Here's how the part is built. I have some questions about the finished solid (model axes, mm). A direction names the side the tool comes from. Coordinates: 2 decimals unless noted, no trailing zeros. Loops run counter-clockwise (first coordinate to the right, second up) from the corner with the lowest first, then second, coordinate; pieces in that order, holes last. Notation, with made-up numbers: (32, 13.5) -> (79, 13.5) arc R11 cw to (79, 26.5) -> close; hole circle Ø9 at (-8, 36.25). An arc over 180 degrees is marked (long way). Answer as a JSON object with one key per item and string values. Group by question number.
1) I want a section at B-B (x = -16). Write out the boundary of the cut face in (y, z).
2) I want a section at A-A (z = 8.5). Write out the boundary of the cut face in (x, y), then the cut area to 3 significant figures.
3) Which directions (+Z, -Z, +X, -X, +Y, -Y) give clear straight access to the entire face, cutting with the end or side of a thin tool? Please do faces 1 (the flat face through (51.619, 2, 5)), 2 (the cylindrical face through (44.05, 1.528, 36.896)).
4) I'm going to push a flat-ended pin straight in: pin 1 (1.9 mm diameter, centred on x = -45.37, z = 38.9, fed in from -Y). Where does the tip first touch, or does it pass through?
5) I want a section at C-C (y = 0.7). Write out the boundary of the cut face in (x, z), then the cut area to 3 significant figures.
6) I need wall thicknesses on probe 1 along X at (y, z) = (2.5, 6.5); probe 2 along Z at (x, y) = (-1, 0.2); probe 3 along Z at (x, y) = (42.5, 1.25). Which ranges of each line are inside material? Lowest first, please. Write a range as [from, to].
7) If we mould it in two halves opening along Z, with no side actions, what happens to faces 3 (the cylindrical face through (40.54, 1.53, -34.79)), 4 (the flat face through (-6, 2, -45.601)), 5 (the flat face through (1, 2, 44.239)), 6 (the flat face through (12, 0, 39))? For each: +Z half, -Z half, draft (parallel to the pull), parting line (faces both ways), or undercut.
```python
from build123d import *

# Parameters (mm, degrees)
SKETCH1_R           = 1.549999996
SKETCH1_R_2         = 1.549999999
SKETCH1_R_3         = 1.550000006
SKETCH1_R_4         = 1.55
BOSS_EXTRUDE1_DEPTH = 3.1


with BuildPart() as part:
    # Sketch1 → Boss-Extrude1 (new body)
    with BuildSketch(Plane(origin=(0, 0, 0), x_dir=(1, 0, 0), z_dir=(0, 1, 0))):
        with BuildLine():
            Line((-39.710740333, 45.601389456), (28.739259425, 45.601389477))
            ThreePointArc((28.739259425, 45.601389477), (44.917862489, 38.899992874), (51.619259444, 22.721389957))
            Line((51.619259444, 22.721389957), (51.619259444, -33.910608927))
            ThreePointArc((51.619259444, -33.910608927), (48.176648434, -41.250850634), (40.639804947, -44.238610519))
            Line((40.639804947, -44.238610519), (-39.710740094, -44.238610544))
            ThreePointArc((-39.710740094, -44.238610544), (-47.488914725, -41.01678516), (-50.710740163, -33.23861055))
            Line((-50.710740163, -33.23861055), (-50.710740163, 34.601389583))
            ThreePointArc((-50.710740163, 34.601389583), (-47.488914793, 42.379564056), (-39.710740333, 45.601389456))
        make_face()
        with Locations(Location((-45.367594445, 40.258243716, 0), (0, 0, 90))):
            Circle(SKETCH1_R, mode=Mode.SUBTRACT)
        with Locations(Location((-45.367594389, -38.895464809, 0), (0, 0, 90))):
            Circle(SKETCH1_R_2, mode=Mode.SUBTRACT)
        with Locations(Location((46.094048666, -39.090808696, 0), (0, 0, 90))):
            Circle(SKETCH1_R_3, mode=Mode.SUBTRACT)
        with Locations(Location((42.796542168, 36.778672508, 0), (0, 0, 90))):
            Circle(SKETCH1_R_4, mode=Mode.SUBTRACT)
        with BuildLine():
            Line((-39.710740331, 39.601389456), (28.739259427, 39.601389477))
            ThreePointArc((28.739259427, 39.601389477), (40.675221825, 34.657352163), (45.619259444, 22.721389891))
            Line((45.619259444, 22.721389891), (45.619259444, -33.691417556))
            ThreePointArc((45.619259444, -33.691417556), (44.011448898, -36.930766758), (40.639804981, -38.238610519))
            Line((40.639804981, -38.238610519), (-39.710740095, -38.238610544))
            ThreePointArc((-39.710740095, -38.238610544), (-43.246274043, -36.774144468), (-44.710740163, -33.238610539))
            Line((-44.710740163, -33.238610539), (-44.710740163, 34.601389583))
            ThreePointArc((-44.710740163, 34.601389583), (-43.246274105, 38.136923369), (-39.710740331, 39.601389456))
        make_face(mode=Mode.SUBTRACT)
    extrude(amount=BOSS_EXTRUDE1_DEPTH)


solid = part.part
```
Determined:
{
 "1": {"outline": "(0, -45.6) -> (3.1, -45.6) -> (3.1, -39.6) -> (0, -39.6) -> close; (0, 38.24) -> (3.1, 38.24) -> (3.1, 44.24) -> (0, 44.24) -> close"},
 "2": {"outline": "(-50.71, 0) -> (-44.71, 0) -> (-44.71, 3.1) -> (-50.71, 3.1) -> close; (45.62, 0) -> (51.62, 0) -> (51.62, 3.1) -> (45.62, 3.1) -> close", "area": "37.2 mm^2"},
 "3": {"face 1": "+Z, -Z, +X, +Y, -Y", "face 2": "+Y, -Y"},
 "4": {"pin 1": "through"},
 "5": {"outline": "(-50.71, -34.6) arc R11 ccw to (-39.71, -45.6) -> (28.74, -45.6) arc R22.88 ccw to (51.62, -22.72) -> (51.62, 33.91) arc R11 ccw to (40.64, 44.24) -> (-39.71, 44.24) arc R11 ccw to (-50.71, 33.24) -> close; hole circle Ø3.1 at (-45.37, -40.26); hole circle Ø3.1 at (-45.37, 38.9); hole (-44.71, -34.6) arc R5 ccw to (-39.71, -39.6) -> (28.74, -39.6) arc R16.88 ccw to (45.62, -22.72) -> (45.62, 33.69) arc R5 ccw to (40.64, 38.24) -> (-39.71, 38.24) arc R5 ccw to (-44.71, 33.24) -> close; hole circle Ø3.1 at (42.8, -36.78); hole circle Ø3.1 at (46.09, 39.09)", "area": "2,020 mm^2"},
 "6": {"probe 1": "[-50.71, -44.71], [45.62, 51.62]", "probe 2": "[-45.6, -39.6], [38.24, 44.24]", "probe 3": "[-41, -38.3], [-35.26, -32.5], [37.88, 44.08]"},
 "7": {"face 3": "undercut", "face 4": "-Z half", "face 5": "+Z half", "face 6": "draft"}
}
